The model under review builds one solid part; all positions refer to its coordinate system, in mm. Coordinates: 2 decimals unless noted, no trailing zeros. Write each loop counter-clockwise with the first axis right and the second up, starting at its lowest first coordinate (ties: lowest second). Pieces come first, ordered by that corner, then holes. Notation, with made-up numbers: (49, -37) - (100, -37) arc R8 ccw to (100, -29) - close; hole circle Ø5 at (31.5, 58). An arc over 180 degrees is marked (long way). Put each result on its own line as item: value.
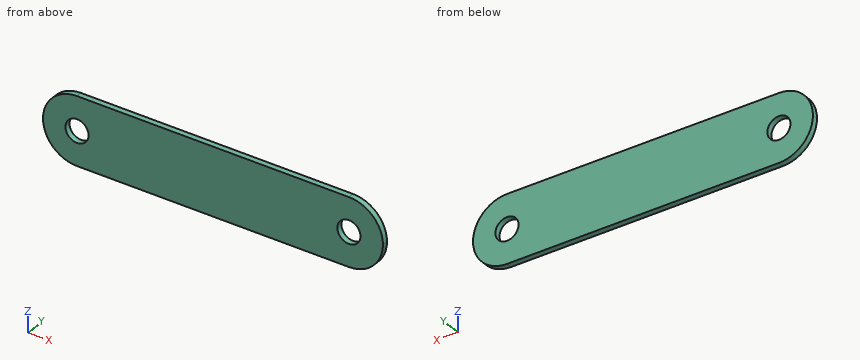
from build123d import *

# Parameters (mm, degrees)
SKETCH1_W                = 50
SKETCH1_H                = 10
BASE_FLANGE1_DEPTH       = 0.86
M3_CLEARANCE_HOLE1_D     = 3.4
M3_CLEARANCE_HOLE1_DEPTH = 1.29
M3_CLEARANCE_HOLE1_TIP   = 1.021463052
FILLET1_R                = 5


# Sheet-metal steps are written as plain solids
with BuildPart() as part:
    # Sketch1 → Base-Flange1 (new body)
    with BuildSketch(Plane(origin=(0, 0, 0), x_dir=(1, 0, 0), z_dir=(0, 1, 0))):
        Rectangle(SKETCH1_W, SKETCH1_H)
    extrude(amount=-BASE_FLANGE1_DEPTH)

    # M3 Clearance Hole1
    with Locations(Plane(origin=(0, 0, 0), x_dir=(1, 0, 0), z_dir=(0, 1, 0))):
        with Locations((-20, 0), (20, 0)):
            Hole(M3_CLEARANCE_HOLE1_D / 2, depth=M3_CLEARANCE_HOLE1_DEPTH)
            with Locations((0, 0, -(M3_CLEARANCE_HOLE1_DEPTH + M3_CLEARANCE_HOLE1_TIP / 2))):  # 118° drill point
                Cone(0, M3_CLEARANCE_HOLE1_D / 2, M3_CLEARANCE_HOLE1_TIP, mode=Mode.SUBTRACT)

    # Fillet1
    fillet1_edges = [part.edges().sort_by_distance(p)[0] for p in [
        (25, -0.43, 5),
        (25, -0.43, -5),
        (-25, -0.43, -5),
        (-25, -0.43, 5),
    ]]
    fillet(fillet1_edges, radius=FILLET1_R - 0.0001)  # a hair under: the kernel refuses the full size


solid = part.part
1. To check wall thickness, follow probe 1 along X at (y, z) = (-0.7, 0.75); probe 2 along Z at (x, y) = (-20, -0.45); probe 3 along X at (y, z) = (-0.8, -1). State the ranges of each line that lie inside material, in increasing order.
Determined:
probe 1: x = -24.94 to -21.53, -18.47 to 18.47, 21.53 to 24.94
probe 2: z = -5 to -1.7, 1.7 to 5
probe 3: x = -24.9 to -21.37, -18.63 to 18.63, 21.37 to 24.9
2. Consider section B-B on z = -1. State the section outline as (x, y) points, plus the area to 3 significant figures.
Determined:
outline: (-24.9, -0.86) - (-21.37, -0.86) - (-21.37, 0) - (-24.9, 0) - close; (-18.63, -0.86) - (18.63, -0.86) - (18.63, 0) - (-18.63, 0) - close; (21.37, -0.86) - (24.9, -0.86) - (24.9, 0) - (21.37, 0) - close
area: 38.1 mm^2
3. Consider section A-A on y = -0.65. Give the number of separate pieces and of enclosed holes in the cut face, plus the area to 3 significant figures.
Determined:
separate pieces: 1
enclosed holes: 2
area: 460 mm^2
4. Consider section C-C on z = -3.5. State the section outline as (x, y) points, plus the area to 3 significant figures.
Determined:
outline: (-23.57, -0.86) - (23.57, -0.86) - (23.57, 0) - (-23.57, 0) - close
area: 40.5 mm^2
